Verification items for this drawing (mm, ordinates from the low corner). A direction names the side the tool comes from. Coordinates: 2 decimals unless noted, no trailing zeros. Write each loop counter-clockwise with the first axis right and the second up, starting at its lowest first coordinate (ties: lowest second). Pieces come first, ordered by that corner, then holes. Notation, with made-up numbers: M -25,66.25 L 10,66.25 A26 cw 10,97.25 Z; hole C 53.25,25 d5. An arc over 180 degrees is marked long. Write each question's results on one line, items separated by ' | '.
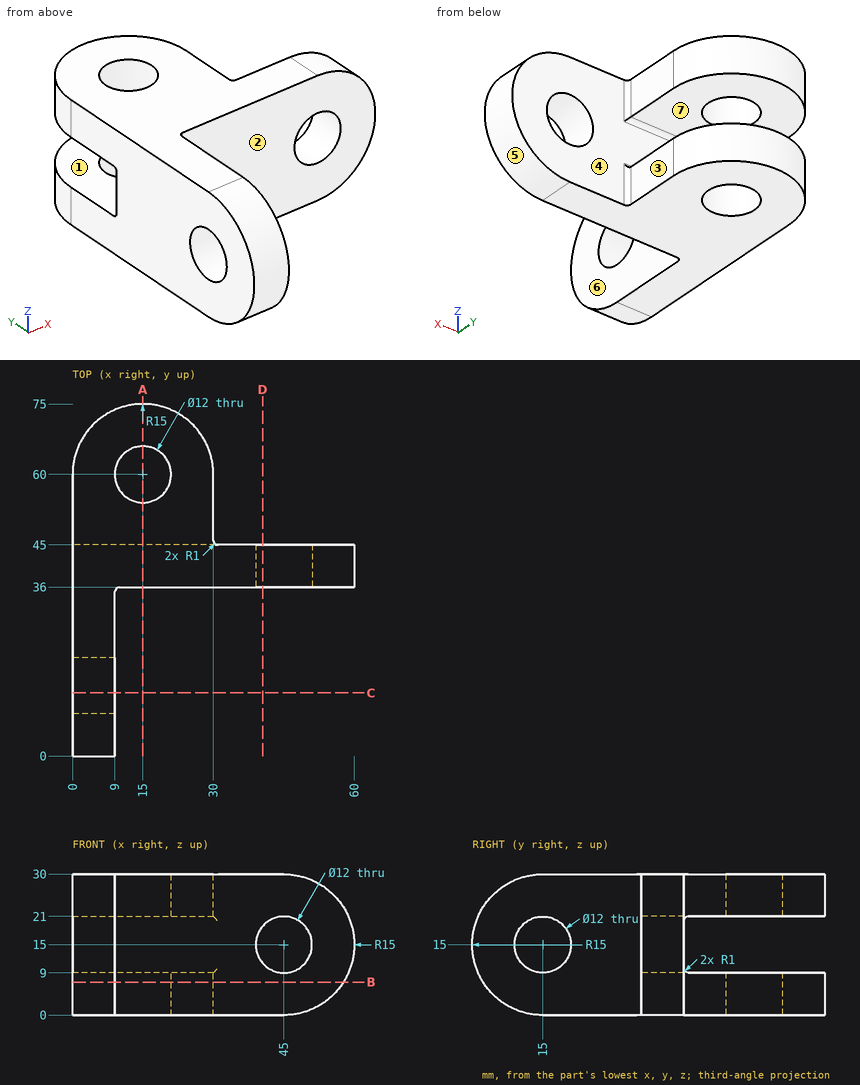
Q1. Sectioned sample at D-D on x = 40.5. Record the cut outline in (y, z), and give its area (3 significant figures).
Geometry check:
outline: M 36,0 L 45,0 L 45,11.03 L 36,11.03 Z; M 36,18.97 L 45,18.97 L 45,30 L 36,30 Z | area: 199 mm2
Q2. Depth check by flat-ended pin: P1, Ø11, axis at x = 15, y = 60, coming from the -Z side; P2, Ø7, axis at y = 53.5, z = 24.5, coming from the +X side; P3, Ø10, axis at x = 32, z = 12, coming from the -Y side; P4, Ø6, axis at y = 49.5, z = 10, coming from the -X side. Enter the tip coordinate at first touch or a pass-through.
Geometry check:
P1: passes through | P2: stops at x = 30 | P3: stops at y = 36 | P4: stops at x = 0
Q3. Scan lines: probe 1 along Y at (x, z) = (5.75, 15); probe 2 along Z at (x, y) = (45, 43); probe 3 along Y at (x, z) = (15, 4). Record each from-to range of solid material in increasing order.
Geometry check:
probe 1: y = 0 to 9, 21 to 45 | probe 2: z = 0 to 9, 21 to 30 | probe 3: y = 36 to 54, 66 to 75
Q4. Sectioned sample at C-C on y = 13.5. Record the cut outline in (x, z), and give its area (3 significant figures).
Geometry check:
outline: M 0,0.08 L 9,0.08 L 9,9.19 L 0,9.19 Z; M 0,20.81 L 9,20.81 L 9,29.92 L 0,29.92 Z | area: 164 mm2
Q5. Mould release check, pull along Z, two halves, no side actions. Record for the marked faces 5, 6 and 7: pulls with the +Z half, pulls with the -Z half, needs draft (parallel to the pull), parting line crosses it, or undercut.
Geometry check:
face 5: parting line crosses it | face 6: needs draft | face 7: undercut
Q6. Access from +Z, -Z, +X, -X, +Y, -Y to the whole of each face (thin tool, end or side, straight path). Record for the marked faces 1, 2, 3 and 4.
Geometry check:
face 1: +X, -X, +Y | face 2: +Z, -Z, +X, -Y | face 3: +Z, -Z, +X, +Y | face 4: +X, +Y
Q7. Sectioned sample at A-A on x = 15. Record the cut outline in (y, z), and give its area (3 significant figures).
Geometry check:
outline: M 36,0 L 54,0 L 54,9 L 46,9 A1 cw 45,10 L 45,20 A1 cw 46,21 L 54,21 L 54,30 L 36,30 Z; M 66,0 L 75,0 L 75,9 L 66,9 Z; M 66,21 L 75,21 L 75,30 L 66,30 Z | area: 594 mm2
Q8. Sectioned sample at B-B on z = 7. Record the cut outline in (x, y), and give its area (3 significant figures).
Geometry check:
outline: M 0,2.31 L 9,2.31 L 9,35 A1 cw 10,36 L 57.69,36 L 57.69,45 L 31,45 A1 cw 30,46 L 30,60 A15 ccw 0,60 Z; hole C 15,60 d12 | area: 1,510 mm2
